```python
from build123d import *

# Parameters (mm, degrees)
SKETCH1_W                = 13
SKETCH1_H                = 13
BOSS_EXTRUDE1_DEPTH      = 3.5
SKETCH2_W                = 22
SKETCH2_H                = 3.7
BOSS_EXTRUDE2_DEPTH      = 3.5
FILLET1_R                = 1.85
SKETCH3_R                = 0.5
CUT_EXTRUDE1_DEPTH       = 3.5
BOSS_EXTRUDE3_DEPTH      = 9
BOSS_EXTRUDE3_DEPTH_BACK = 3.5
SKETCH4_R                = 6.75
SKETCH5_R                = 0.5
CUT_EXTRUDE2_DEPTH       = 9
SKETCH6_R                = 6
CUT_EXTRUDE3_DEPTH       = 9


with BuildPart() as part:
    # Sketch1 → Boss-Extrude1 (new body)
    with BuildSketch(Plane.XY):
        Rectangle(SKETCH1_W, SKETCH1_H)
    extrude(amount=BOSS_EXTRUDE1_DEPTH)

    # Sketch2 → Boss-Extrude2 (add)
    with BuildSketch(Plane.XY.offset(3.5)):
        Rectangle(SKETCH2_W, SKETCH2_H)
    extrude(amount=-BOSS_EXTRUDE2_DEPTH)

    # Fillet1
    fillet1_edges = [part.edges().sort_by_distance(p)[0] for p in [
        (11, -1.85, 1.75),
        (11, 1.85, 1.75),
        (-11, -1.85, 1.75),
        (-11, 1.85, 1.75),
    ]]
    fillet(fillet1_edges, radius=FILLET1_R - 0.0001)  # a hair under: the kernel refuses the full size

    # Sketch3 → Cut-Extrude1 (cut)
    with BuildSketch(Plane.XY.offset(3.5)):
        with Locations((-9, 0)):
            Circle(SKETCH3_R)
        with Locations((9, 0)):
            Circle(SKETCH3_R)
    extrude(amount=-CUT_EXTRUDE1_DEPTH, mode=Mode.SUBTRACT)

    # Sketch4 → Boss-Extrude3 (add, two sides: drawn at the far end of the back side and taken through both)
    with BuildSketch(Plane.XY.offset(3.5).offset(-BOSS_EXTRUDE3_DEPTH_BACK)):
        Circle(SKETCH4_R)
    extrude(amount=BOSS_EXTRUDE3_DEPTH + BOSS_EXTRUDE3_DEPTH_BACK)

    # Sketch5 → Cut-Extrude2 (cut)
    with BuildSketch(Plane.XY.offset(12.5)):
        with Locations((0, 7)):
            Circle(SKETCH5_R)
        with Locations((1.324758711, 6.873500881)):
            Circle(SKETCH5_R)
        with Locations((2.60163719, 6.498575531)):
            Circle(SKETCH5_R)
        with Locations((3.784485722, 5.88877473)):
            Circle(SKETCH5_R)
        with Locations((4.83055308, 5.066138267)):
            Circle(SKETCH5_R)
        with Locations((5.702031664, 4.060398367)):
            Circle(SKETCH5_R)
        with Locations((6.367423967, 2.907905091)):
            Circle(SKETCH5_R)
        with Locations((6.802680978, 1.650312549)):
            Circle(SKETCH5_R)
        with Locations((6.992071374, 0.333073411)):
            Circle(SKETCH5_R)
        with Locations((6.928750093, -0.996203868)):
            Circle(SKETCH5_R)
        with Locations((6.615005731, -2.289475743)):
            Circle(SKETCH5_R)
        with Locations((6.062177826, -3.5)):
            Circle(SKETCH5_R)
        with Locations((5.29024702, -4.584025138)):
            Circle(SKETCH5_R)
        with Locations((4.327112904, -5.502371663)):
            Circle(SKETCH5_R)
        with Locations((3.207585652, -6.221848141)):
            Circle(SKETCH5_R)
        with Locations((1.972127898, -6.716450815)):
            Circle(SKETCH5_R)
        with Locations((0.665392303, -6.968303458)):
            Circle(SKETCH5_R)
        with Locations((-0.665392303, -6.968303458)):
            Circle(SKETCH5_R)
        with Locations((-1.972127898, -6.716450815)):
            Circle(SKETCH5_R)
        with Locations((-3.207585652, -6.221848141)):
            Circle(SKETCH5_R)
        with Locations((-4.327112904, -5.502371663)):
            Circle(SKETCH5_R)
        with Locations((-5.29024702, -4.584025138)):
            Circle(SKETCH5_R)
        with Locations((-6.062177826, -3.5)):
            Circle(SKETCH5_R)
        with Locations((-6.615005731, -2.289475743)):
            Circle(SKETCH5_R)
        with Locations((-6.928750093, -0.996203868)):
            Circle(SKETCH5_R)
        with Locations((-6.992071374, 0.333073411)):
            Circle(SKETCH5_R)
        with Locations((-6.802680978, 1.650312549)):
            Circle(SKETCH5_R)
        with Locations((-6.367423967, 2.907905091)):
            Circle(SKETCH5_R)
        with Locations((-5.702031664, 4.060398367)):
            Circle(SKETCH5_R)
        with Locations((-4.83055308, 5.066138267)):
            Circle(SKETCH5_R)
        with Locations((-3.784485722, 5.88877473)):
            Circle(SKETCH5_R)
        with Locations((-2.60163719, 6.498575531)):
            Circle(SKETCH5_R)
        with Locations((-1.324758711, 6.873500881)):
            Circle(SKETCH5_R)
    extrude(amount=-CUT_EXTRUDE2_DEPTH, mode=Mode.SUBTRACT)

    # Sketch6 → Cut-Extrude3 (cut)
    with BuildSketch(Plane.XY.offset(12.5)):
        Circle(SKETCH6_R)
    extrude(amount=-CUT_EXTRUDE3_DEPTH, mode=Mode.SUBTRACT)


solid = part.part
```
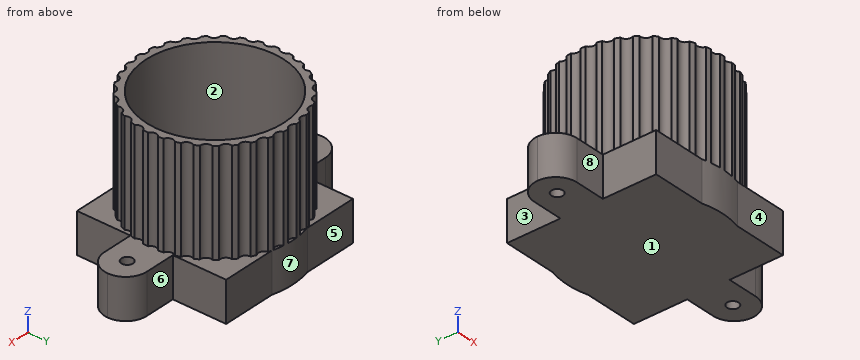
For this review, take the finished solid that the model builds, in its own axes (mm). Face numbers are marked on the shaded views. A direction names the side the tool comes from. Coordinates: 2 decimals unless noted, no trailing zeros. Write each loop counter-clockwise with the first axis right and the second up, starting at its lowest first coordinate (ties: lowest second). Pieces come first, ordered by that corner, then holes. Notation, with made-up numbers: (20.25, -38.75) -> (70.25, -38.75) arc R18 cw to (70.25, -22.75) -> close; hole circle Ø5 at (-22, -25). An arc over 180 degrees is marked (long way). Put each result on its own line as item: value.
Q1. The part is to be moulded in two halves that separate along X. For the marked faces 1, 2 and 3, say which applies: +X half, -X half, draft (parallel to the pull), parting line (faces both ways), or undercut.
From the geometry:
face 1: draft
face 2: undercut
face 3: -X half
Q2. Clearance check with flat-ended pins moving along their axes: pin 1 Ø3 at (y, z) = (2, 5.5) entering from -X; pin 2 Ø1.8 at (y, z) = (-5, 1) entering from +X; pin 3 Ø4 at (y, z) = (5, 1.5) entering from -X. State where each tip first meets the part, or that it passes through.
From the geometry:
pin 1: stops at x = -6.71
pin 2: stops at x = 6.5
pin 3: stops at x = -6.5
Q3. Take a section at B-B, the plane y = 0.25. State the section outline as (x, z) points.
From the geometry:
outline: (-10.98, 0) -> (-9.43, 0) -> (-9.43, 3.5) -> (-10.98, 3.5) -> close; (-8.57, 0) -> (8.57, 0) -> (8.57, 3.5) -> (6.5, 3.5) -> (6.5, 12.5) -> (5.99, 12.5) -> (5.99, 3.5) -> (-5.99, 3.5) -> (-5.99, 12.5) -> (-6.5, 12.5) -> (-6.5, 3.5) -> (-8.57, 3.5) -> close; (9.43, 0) -> (10.98, 0) -> (10.98, 3.5) -> (9.43, 3.5) -> close
Q4. Tool access review of the marked faces 4, 5, 6, 7 and 8: name each direction out of +Z, -Z, +X, -X, +Y, -Y from which nothing blocks a thin tool from reaching the whole face with its end or side.
From the geometry:
face 4: +Z, -Z, +X, -Y
face 5: +Z, -Z, -X, +Y
face 6: +Z, -Z, +X, +Y
face 7: +Z, +Y
face 8: +Z, -Z, -X, -Y
Q5. Wall thickness on L1, parallel to Y at x = -9, z = 1.3; L2, parallel to Z at x = -0.5, y = 1; L3, parallel to Y at x = -5.5, z = 3.25: over which ranges is each line inside the solid? List them lowest first.
From the geometry:
L1: y = -1.85 to -0.5, 0.5 to 1.85
L2: z = 0 to 3.5
L3: y = -6.5 to 6.5
Q6. Take a section at A-A, the plane z = 1.5. Count the separate pieces of the cut face and the enclosed holes in it, then the cut area to 3 significant figures.
From the geometry:
separate pieces: 1
enclosed holes: 2
area: 199 mm2
